Check sheet for the modelled part. Datum: model origin and axes. Units: mm. Face numbers are marked on the shaded views. A direction names the side the tool comes from. Give positions to 0.01 mm unless a question says otherwise; leave off trailing zeros. Order: outer loops, then holes, each group sorted by start corner. A loop starts at its lowest first (then second) coordinate and runs counter-clockwise, first axis right, second up.
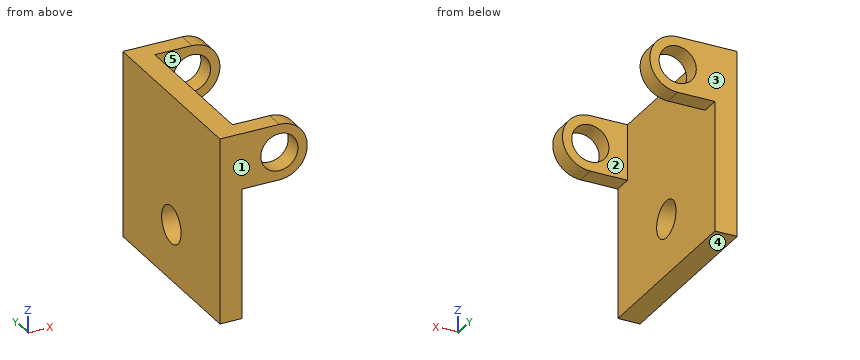
from build123d import *

# Parameters (mm, degrees)
F1_DEPTH = 10
F2_W     = 100
F2_H     = 100
F3_DEPTH = 12
F5_DEPTH = 10
F7_D     = 20
F9_D     = 20


with BuildPart() as f1:
    # F0 (on Front) → F1 (new body)
    with BuildSketch(Plane.XZ):
        with BuildLine():
            Line((0, 30), (0, 0))
            Line((0, 0), (20, 0))
            Line((20, 0), (20, 10))
            ThreePointArc((20, 10), (15, 15), (20, 20))
            Line((20, 20), (20, 30))
            Line((20, 30), (0, 30))
        make_face()
        with BuildLine():
            Line((20, 10), (20, 0))
            ThreePointArc((20, 0), (35, 15), (20, 30))
            Line((20, 30), (20, 20))
            ThreePointArc((20, 20), (23.535534, 18.535534), (25, 15))
            ThreePointArc((25, 15), (23.535534, 11.464466), (20, 10))
        make_face()
    extrude(amount=F1_DEPTH)

    # F2 (on Right) → F3 (join)
    with BuildSketch(Plane.YZ):
        with Locations((-50, -20)):
            Rectangle(F2_W, F2_H)
    extrude(amount=-F3_DEPTH)

    # F4 (on face) → F5 (join)
    with BuildSketch(Plane.XZ.offset(100)):
        with BuildLine():
            Line((0, 30), (0, 0))
            Line((0, 0), (20, 0))
            Line((20, 0), (20, 10))
            ThreePointArc((20, 10), (15, 15), (20, 20))
            Line((20, 20), (20, 30))
            Line((20, 30), (0, 30))
        make_face()
        with BuildLine():
            Line((20, 10), (20, 0))
            ThreePointArc((20, 0), (35, 15), (20, 30))
            Line((20, 30), (20, 20))
            ThreePointArc((20, 20), (23.535534, 18.535534), (25, 15))
            ThreePointArc((25, 15), (23.535534, 11.464466), (20, 10))
        make_face()
    extrude(amount=-F5_DEPTH)

    # F7 (through all)
    with Locations(Plane(origin=(-12, 0, 0), x_dir=(0, -1, 0), z_dir=(-1, 0, 0))):
        with Locations((50, -40)):
            Hole(F7_D / 2)

    # F9 (through all)
    with Locations(Plane.XZ.offset(100)):
        with Locations((20, 15)):
            Hole(F9_D / 2)


solid = f1.part
1) Section check B-B, the plane x = -5.5. Record the cut outline in (y, z).
Recorded:
outline: (-100, -70) - (0, -70) - (0, 30) - (-100, 30) - close; hole circle Ø20 at (-50, -40)
2) Set-up check for the marked faces 1 and 2: record each of +Z, -Z, +X, -X, +Y, -Y from which the full face is reachable in a straight line by a thin tool's end or side.
Recorded:
face 1: +Z, -Z, +X, -X, -Y
face 2: +Z, -Z, +X
3) Material ranges on L1, parallel to Z at x = -6.25, y = -50; L2, parallel to X at y = -27, z = -16; L3, parallel to Z at x = 20, y = -96, recorded low to high.
Recorded:
L1: z = -70 to -50, -30 to 30
L2: x = -12 to 0
L3: z = 0 to 5, 25 to 30
4) Section check D-D, the plane z = 15. Record the cut outline in (x, y), then the cut area to 3 significant figures.
Recorded:
outline: (-12, -100) - (10, -100) - (10, -90) - (0, -90) - (0, -10) - (10, -10) - (10, 0) - (-12, 0) - close; (30, -100) - (35, -100) - (35, -90) - (30, -90) - close; (30, -10) - (35, -10) - (35, 0) - (30, 0) - close
area: 1,500 mm2
5) Section check A-A, the plane z = -40. Record the cut outline in (x, y), then the cut area to 3 significant figures.
Recorded:
outline: (-12, -100) - (0, -100) - (0, -60) - (-12, -60) - close; (-12, -40) - (0, -40) - (0, 0) - (-12, 0) - close
area: 960 mm2
6) Section check C-C, the plane y = -44. Record the cut outline in (x, z).
Recorded:
outline: (-12, -70) - (0, -70) - (0, -48) - (-12, -48) - close; (-12, -32) - (0, -32) - (0, 30) - (-12, 30) - close
7) Depth check by flat-ended pin: pin 1 Ø8 at (x, y) = (12, -97) entering from -Z; pin 2 Ø18 at (y, z) = (-50, -40) entering from +X; pin 3 Ø8 at (y, z) = (-69.5, -31) entering from +X. Enter the tip coordinate at first touch or a pass-through.
Recorded:
pin 1: stops at z = 0
pin 2: passes through
pin 3: stops at x = 0
8) Draft check along Y on the marked faces 3, 4 and 5. Enter one of: +Y half, -Y half, draft (parallel to the pull), parting line (faces both ways), or undercut.
Recorded:
face 3: +Y half
face 4: draft
face 5: undercut
